Read the model definition and answer for the solid it produces. Units are mm, in the model's axes. Coordinates: 2 decimals unless noted, no trailing zeros. Loops run counter-clockwise (first coordinate to the right, second up) from the corner with the lowest first, then second, coordinate; pieces in that order, holes last. Notation, with made-up numbers: M 60,-13 L 103,-13 A34 cw 103,25 Z; hole C 30,76 d8. An arc over 180 degrees is marked long. Put each result on its own line as item: value.
from build123d import *

# Parameters (mm, degrees)
SKETCH1_W           = 60
SKETCH1_H           = 8
SKETCH1_R           = 2.58
SKETCH1_R_2         = 2.59
BOSS_EXTRUDE1_DEPTH = 3
REDONDEO2_R         = 4


with BuildPart() as part:
    # Sketch1 → Boss-Extrude1 (new body)
    with BuildSketch(Plane(origin=(0, 0, 0), x_dir=(1, 0, 0), z_dir=(0, 1, 0))):
        Rectangle(SKETCH1_W, SKETCH1_H)
        with Locations(Location((-25, 0, 0), (0, 0, 270))):
            Circle(SKETCH1_R, mode=Mode.SUBTRACT)
        with Locations(Location((25, 0, 0), (0, 0, 270))):
            Circle(SKETCH1_R_2, mode=Mode.SUBTRACT)
    extrude(amount=BOSS_EXTRUDE1_DEPTH)

    # Redondeo2
    redondeo2_edges = [part.edges().sort_by_distance(p)[0] for p in [
        (30, 1.5, -4),
        (30, 1.5, 4),
        (-30, 1.5, -4),
        (-30, 1.5, 4),
    ]]
    fillet(redondeo2_edges, radius=REDONDEO2_R - 0.0001)  # a hair under: the kernel refuses the full size


solid = part.part
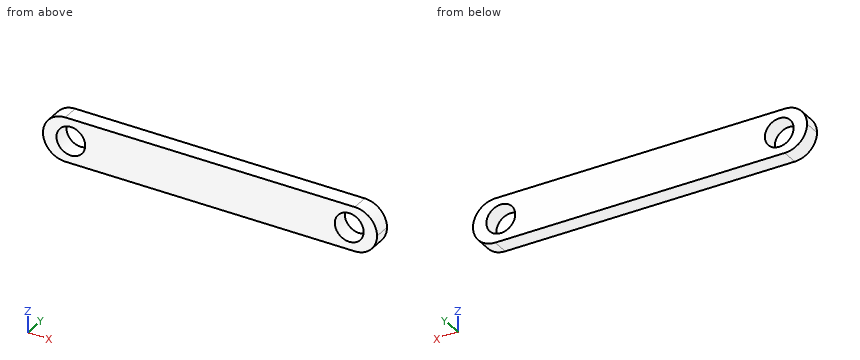
1) Find section B-B, the plane z = 1. Write down the section's boundary in (x, y).
Answer list:
outline: M -29.87,0 L -27.38,0 L -27.38,3 L -29.87,3 Z; M -22.62,0 L 22.61,0 L 22.61,3 L -22.62,3 Z; M 27.39,0 L 29.87,0 L 29.87,3 L 27.39,3 Z
2) Find section C-C, the plane y = 1.7. Count the separate pieces of the cut face and the enclosed holes in it, plus the area to 3 significant figures.
Answer list:
separate pieces: 1
enclosed holes: 2
area: 424 mm^2
3) Find section D-D, the plane x = -25. Write down the section's boundary in (y, z).
Answer list:
outline: M 0,-4 L 3,-4 L 3,-2.58 L 0,-2.58 Z; M 0,2.58 L 3,2.58 L 3,4 L 0,4 Z
4) Given pin 1 Ø1 at (x, z) = (6, -1) entering from -Y, flat-ended and moving along its own axis, determine where the tip first touches the part or whether it passes through.
Answer list:
pin 1: stops at y = 0
5) Straight lines are drawn through the part: line 1 (X direction, y = 1, z = 0); line 2 (X direction, y = 1.6, z = 1.25); line 3 (Z direction, x = 24, y = 1.05). For each, find the intervals that lie inside material, in ascending order. Write a range as [from, to].
Answer list:
line 1: x = [-30, -27.58], [-22.42, 22.41], [27.59, 30]
line 2: x = [-29.8, -27.26], [-22.74, 22.73], [27.27, 29.8]
line 3: z = [-4, -2.39], [2.39, 4]
6) Find section A-A, the plane x = 25. Write down the section's boundary in (y, z), plus the area to 3 significant figures.
Answer list:
outline: M 0,-4 L 3,-4 L 3,-2.59 L 0,-2.59 Z; M 0,2.59 L 3,2.59 L 3,4 L 0,4 Z
area: 8.46 mm^2
